Geometry: final body of the model. Coordinates: model frame, mm. A direction names the side the tool comes from. Coordinates: 2 decimals unless noted, no trailing zeros. Order: outer loops, then holes, each group sorted by start corner. A loop starts at its lowest first (then second) coordinate and runs counter-clockwise, first axis right, second up. Notation, with made-up numbers: M 68.5,70.5 L 123.5,70.5 A25 cw 123.5,108.5 Z; hole C -31,14 d2. An arc over 180 degrees is marked long. Write item = value, one per line.
from build123d import *

# Parameters (mm, degrees)
F3_DEPTH = 12.5


with BuildPart() as f1:
    # F0 (on Front) → F1 (revolve)
    with BuildSketch(Plane.XZ):
        Polygon((2.75, 9.6877501001), (1.8, 10), (1.8, 0), (2.75, 0), (2.75, 1.6877501001), (3, 1.6877501001), (2.75, 3.6877501001), (2.75, 5.6877501001), (3, 5.6877501001), (2.75, 7.6877501001), align=None)
    revolve(axis=Axis((0, 0, 0.3669395117), (0, 0, -1)))

    # F2 (on Front) → F3 (cut, symmetric)
    with BuildSketch(Plane.XZ):
        Polygon((0.5, 10), (-0.5, 10), (-0.5, 1.5), (0, 1.5), (0.5, 1.5), align=None)
    extrude(amount=F3_DEPTH, both=True, mode=Mode.SUBTRACT)


solid = f1.part
1) Section A-A, the plane x = 0. Return loops of the section in (y, z).
Numbers:
outline = M -2.75,0 L -1.8,0 L -1.8,1.5 L -2.75,1.5 Z; M 1.8,0 L 2.75,0 L 2.75,1.5 L 1.8,1.5 Z
2) Line query: L1, parallel to X at y = 0, z = 5; L2, parallel to X at y = 1.8, z = 7; L3, parallel to Y at x = -1, z = 3.75. Output: solid intervals per line, ascending.
Numbers:
L1 = -2.75 to -1.8, 1.8 to 2.75
L2 = -2.19 to -0.5, 0.5 to 2.19
L3 = -2.56 to -1.5, 1.5 to 2.56
3) Mould query, pull axis X, two halves, no side actions, for faces 4 (the face through (2.75, 0.05, 8.7)), 5 (the face through (0.5, -2, 6)), 6 (the face through (-2.75, -0.05, 8.7)). Classes: pulls with the +X half, pulls with the -X half, needs draft (parallel to the pull), parting line crosses it, or undercut.
Numbers:
face_4 = pulls with the +X half
face_5 = undercut
face_6 = pulls with the -X half
4) Section B-B, the plane y = 0. Return loops of the section in (x, z), and give its area (3 significant figures).
Numbers:
outline = M -3,1.69 L -2.75,1.69 L -2.75,0 L -1.8,0 L -1.8,10 L -2.75,9.69 L -2.75,7.69 L -3,5.69 L -2.75,5.69 L -2.75,3.69 Z; M 1.8,0 L 2.75,0 L 2.75,1.69 L 3,1.69 L 2.75,3.69 L 2.75,5.69 L 3,5.69 L 2.75,7.69 L 2.75,9.69 L 1.8,10 Z
area = 19.7 mm²
5) Set-up query: faces 1 (the face through (0, -2, 1.5)), 2 (the face through (-2.75, -0.05, 4.7)), 3 (the face through (2.873, 0.056, 2.702)). Return all of +Z, -Z, +X, -X, +Y, -Y with unobstructed straight access to the full face (end or side cutting, diameter ignored); none if empty.
Numbers:
face_1 = +Z, +Y, -Y
face_2 = -X
face_3 = +X
6) Pin query (flat end, axial travel): pin 1 (1.5 mm diameter, centred on x = 0.5, z = 3.5, fed in from +Y); pin 2 (2 mm diameter, centred on x = 2, y = -1, fed in from -Z); pin 3 (1.4 mm diameter, centred on y = 2.5, z = 7, fed in from -X); pin 4 (0.5 mm diameter, centred on x = 0, y = -2, fed in from +Z). Return the tip coordinate at first contact, or that it passes through.
Numbers:
pin_1 = 2.82
pin_2 = 0
pin_3 = -2.2
pin_4 = 1.5
7) Section C-C, the plane z = 4.25. Return loops of the section in (x, y), and give its area (3 significant figures).
Numbers:
outline = M -0.5,-2.7 L -0.5,-1.73 A1.8 cw -0.5,1.73 L -0.5,2.7 A2.75 ccw Z; M 0.5,-2.7 A2.75 ccw 0.5,2.7 L 0.5,1.73 A1.8 cw 0.5,-1.73 Z
area = 11.7 mm²
